```python
from build123d import *

# Parameters (mm, degrees)
SKETCH1_R           = 4.7
BOSS_EXTRUDE1_DEPTH = 45
SKETCH2_R           = 6.75
BOSS_EXTRUDE2_DEPTH = 2
CHAMFER2_SIZE       = 0.4
CHAMFER3_SIZE       = 0.4


with BuildPart() as part:
    # Sketch1 → Boss-Extrude1 (new body)
    with BuildSketch(Plane(origin=(0, 0, 0), x_dir=(1, 0, 0), z_dir=(0, 1, 0))):
        Circle(SKETCH1_R)
    extrude(amount=BOSS_EXTRUDE1_DEPTH)

    # Sketch2 → Boss-Extrude2 (add)
    with BuildSketch(Plane(origin=(0, 45, 0), x_dir=(1, 0, 0), z_dir=(0, 1, 0))):
        Circle(SKETCH2_R)
    extrude(amount=-BOSS_EXTRUDE2_DEPTH)

    # Chamfer2
    chamfer2_edges = [part.edges().sort_by_distance(p)[0] for p in [
        (-6.75, 43, 0),
        (-6.75, 45, 0),
    ]]
    chamfer(chamfer2_edges, length=CHAMFER2_SIZE)

    # Chamfer3
    chamfer3_edges = [part.edges().sort_by_distance(p)[0] for p in [
        (-4.7, 0, 0),
    ]]
    chamfer(chamfer3_edges, length=CHAMFER3_SIZE)


solid = part.part
```
Geometry: final body of the model. Coordinates: model frame, mm. A direction names the side the tool comes from. Round coordinates to 2 decimals unless told otherwise and drop trailing zeros. Write each loop counter-clockwise with the first axis right and the second up, starting at its lowest first coordinate (ties: lowest second). Pieces come first, ordered by that corner, then holes. Notation, with made-up numbers: M -7.5,-25 L 13.5,-25 A18 cw 13.5,6 Z; hole C 53.5,76.5 d3. An arc over 180 degrees is marked long. Answer in a Markdown table with one row per item. Add a question column.
(1) Cut plane A-A, the plane x = 0. Return the cut outline in (y, z), then the cut area to 3 significant figures.
(2) Cut plane B-B, the plane z = 0. Return the cut outline in (x, y), then the cut area to 3 significant figures.
(3) Reachability of faces 1 (the face through (0, 43, -5)), 2 (the face through (0, 0, 0)) from +Z, -Z, +X, -X, +Y, -Y: full face, straight path, thin tool, end or side. Return the list, or none.
(4) Contact query for flat-ended pins moving along their axis: pin 1 (4 mm diameter, centred on y = 40, z = 0, fed in from +X); pin 2 (1.5 mm diameter, centred on x = -1.5, y = 31, fed in from -Z); pin 3 (2 mm diameter, centred on x = 0, y = 37.5, fed in from +Z). Output: stop coordinate, or through.
(5) Ray query, L1, parallel to Y at x = 5.5, z = 2.5; L2, parallel to Z at x = 0.25, y = 38; L3, parallel to X at y = 27, z = -3.5. Return the intervals inside material, ascending.
(6) Cut plane C-C, the plane y = 20. Return the cut outline in (x, z).
Established:
| question | item | result |
|---|---|---|
| 1 | outline | M 0,-4.3 L 0.4,-4.7 L 43,-4.7 L 43,-6.35 L 43.4,-6.75 L 44.6,-6.75 L 45,-6.35 L 45,6.35 L 44.6,6.75 L 43.4,6.75 L 43,6.35 L 43,4.7 L 0.4,4.7 L 0,4.3 Z |
| 1 | area | 431 mm² |
| 2 | outline | M -6.75,43.4 L -6.35,43 L -4.7,43 L -4.7,0.4 L -4.3,0 L 4.3,0 L 4.7,0.4 L 4.7,43 L 6.35,43 L 6.75,43.4 L 6.75,44.6 L 6.35,45 L -6.35,45 L -6.75,44.6 Z |
| 2 | area | 431 mm² |
| 3 | face 1 | -Y |
| 3 | face 2 | +Z, -Z, +X, -X, -Y |
| 4 | pin 1 | x = 4.7 |
| 4 | pin 2 | z = -4.64 |
| 4 | pin 3 | z = 4.7 |
| 5 | L1 | 43 to 45 |
| 5 | L2 | -4.69 to 4.69 |
| 5 | L3 | -3.14 to 3.14 |
| 6 | outline | C 0,0 d9.4 |
